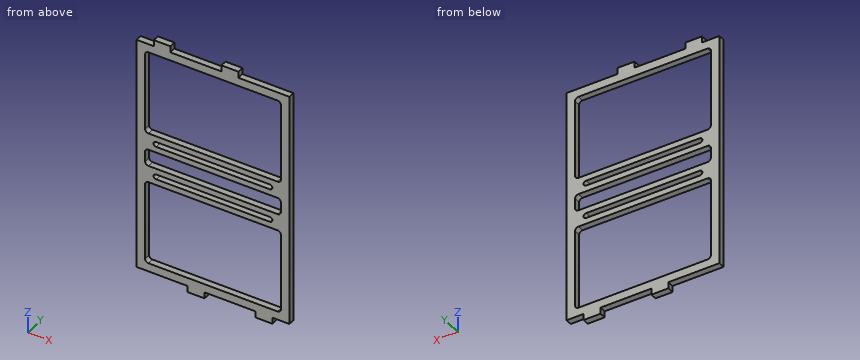
from build123d import *

# Parameters (mm, degrees)
SKETCH1_W           = 114.3
SKETCH1_H           = 177.8
SKETCH1_W_2         = 101.6
SKETCH1_H_2         = 165.1
BOSS_EXTRUDE1_DEPTH = 4.7625
SKETCH2_W           = 12.38677804
SKETCH2_H           = 4.7625
SKETCH2_W_2         = 12.7
BOSS_EXTRUDE2_DEPTH = 4.7625
SKETCH3_W           = 12.7
SKETCH3_H           = 4.7625
BOSS_EXTRUDE3_DEPTH = 4.7625
SKETCH7_W           = 114.3
SKETCH7_H           = 12.7
SKETCH7_W_2         = 88.9
SKETCH7_H_2         = 3.81
BOSS_EXTRUDE5_DEPTH = 4.7625
FILLET1_R           = 2.54
FILLET2_R           = 1.905


with BuildPart() as part:
    # Sketch1 → Boss-Extrude1 (new body)
    with BuildSketch(Plane(origin=(0, 0, 0), x_dir=(1, 0, 0), z_dir=(0, 1, 0))):
        Rectangle(SKETCH1_W, SKETCH1_H)
        Rectangle(SKETCH1_W_2, SKETCH1_H_2, mode=Mode.SUBTRACT)
    extrude(amount=BOSS_EXTRUDE1_DEPTH)

    # Sketch2 → Boss-Extrude2 (add)
    with BuildSketch(Plane.XY.offset(88.9)):
        with Locations((-38.1, 2.38125)):
            Rectangle(SKETCH2_W, SKETCH2_H)
        with Locations((12.7, 2.38125)):
            Rectangle(SKETCH2_W_2, SKETCH2_H)
    extrude(amount=BOSS_EXTRUDE2_DEPTH)

    # Sketch3 → Boss-Extrude3 (add)
    with BuildSketch(Plane(origin=(0, 0, -88.9), x_dir=(-1, 0, 0), z_dir=(0, 0, -1))):
        with Locations((-38.1, 2.38125)):
            Rectangle(SKETCH3_W, SKETCH3_H)
        with Locations((12.7, 2.38125)):
            Rectangle(SKETCH3_W, SKETCH3_H)
    extrude(amount=BOSS_EXTRUDE3_DEPTH)

    # Sketch7 → Boss-Extrude5 (add)
    # profile 1 of 2: a face of its own
    with BuildSketch(Plane(origin=(0, 4.7625, 0), x_dir=(1, 0, 0), z_dir=(0, 1, 0))):
        with Locations((0, 12.7)):
            Rectangle(SKETCH7_W, SKETCH7_H)
        with Locations((0, 12.7)):
            Rectangle(SKETCH7_W_2, SKETCH7_H_2, mode=Mode.SUBTRACT)
    # profile 2 of 2: a face of its own
    with BuildSketch(Plane(origin=(0, 4.7625, 0), x_dir=(1, 0, 0), z_dir=(0, 1, 0))):
        with Locations((0, -12.7)):
            Rectangle(SKETCH7_W, SKETCH7_H)
        with Locations((0, -12.7)):
            Rectangle(SKETCH7_W_2, SKETCH7_H_2, mode=Mode.SUBTRACT)
    extrude(amount=-BOSS_EXTRUDE5_DEPTH)

    # Fillet1
    fillet1_edges = [part.edges().sort_by_distance(p)[0] for p in [
        (50.8, 2.38125, -19.05),
        (50.8, 2.38125, -6.35),
        (-50.8, 2.38125, 19.05),
        (-50.8, 2.38125, 6.35),
        (50.8, 2.38125, 6.35),
        (50.8, 2.38125, 19.05),
        (50.8, 2.38125, 82.55),
        (50.8, 2.38125, -82.55),
        (-50.8, 2.38125, -82.55),
        (-50.8, 2.38125, 82.55),
        (-50.8, 2.38125, -6.35),
        (-50.8, 2.38125, -19.05),
    ]]
    fillet(fillet1_edges, radius=FILLET1_R)

    # Fillet2
    fillet2_edges = [part.edges().sort_by_distance(p)[0] for p in [
        (-44.45, 2.38125, -10.795),
        (-44.45, 2.38125, -14.605),
        (44.45, 2.38125, -10.795),
        (44.45, 2.38125, -14.605),
        (44.45, 2.38125, 14.605),
        (44.45, 2.38125, 10.795),
        (-44.45, 2.38125, 14.605),
        (-44.45, 2.38125, 10.795),
    ]]
    fillet(fillet2_edges, radius=FILLET2_R - 0.0001)  # a hair under: the kernel refuses the full size


solid = part.part
Here's how the part is built. I have some questions about the finished solid (model axes, mm). Coordinates: 2 decimals unless noted, no trailing zeros. Order: outer loops, then holes, each group sorted by start corner. A loop starts at its lowest first (then second) coordinate and runs counter-clockwise, first axis right, second up.
Item 1: For P1, Ø2.5, axis at x = -22, y = 2, coming from the -Z side; P2, Ø2.5, axis at x = -8.5, y = 3, coming from the +Z side, each with a flat end and sliding along its axis, tell me the tip position at first contact or that it passes through.
Result sheet:
P1: stops at z = -88.9
P2: stops at z = 88.9
Item 2: I need wall thicknesses on line 1 (Z direction, x = -30.5, y = 1.75) (3 decimals); line 2 (Z direction, x = 44, y = 3.6); line 3 (X direction, y = 0.85, z = -50). Which ranges of each line are inside material? Lowest first, please.
Result sheet:
line 1: z = -88.9 to -82.55, -19.05 to -14.605, -10.795 to -6.35, 6.35 to 10.795, 14.605 to 19.05, 82.55 to 88.9
line 2: z = -93.66 to -82.55, -19.05 to -13.93, -11.47 to -6.35, 6.35 to 11.47, 13.93 to 19.05, 82.55 to 88.9
line 3: x = -57.15 to -50.8, 50.8 to 57.15
Item 3: If we section it at B-B on z = -43.5: List the corners of the cut face in (x, y) for me, plus the area to 3 significant figures.
Result sheet:
outline: (-57.15, 0) - (-50.8, 0) - (-50.8, 4.76) - (-57.15, 4.76) - close; (50.8, 0) - (57.15, 0) - (57.15, 4.76) - (50.8, 4.76) - close
area: 60.5 mm2
Item 4: If we section it at A-A on x = 14: State how many separate pieces and enclosed holes the cut face has, plus the area to 3 significant figures.
Result sheet:
separate pieces: 6
enclosed holes: 0
area: 168 mm2
